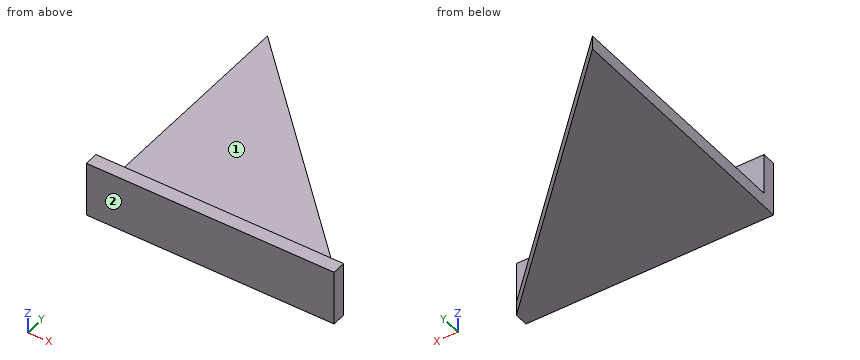
from build123d import *

# Parameters (mm, degrees)
F0_W     = 228.6
F0_H     = 50.8
F1_DEPTH = 12.7
F2_W     = 228.6
F2_H     = 12.7
F3_DEPTH = 228.6
F5_DEPTH = 25.4


with BuildPart() as f1:
    # F0 (on Front) → F1 (new body)
    with BuildSketch(Plane.XZ):
        Rectangle(F0_W, F0_H)
    extrude(amount=F1_DEPTH)

    # F2 (on face) → F3 (join)
    with BuildSketch(Plane(origin=(0, 0, 0), x_dir=(-1, 0, 0), z_dir=(0, 1, 0))):
        with Locations((0, -19.05)):
            Rectangle(F2_W, F2_H)
    extrude(amount=F3_DEPTH)

    # F4 (on face) → F5 (cut)
    with BuildSketch(Plane.XY.offset(-12.7)):
        Polygon((114.3, 228.6), (-114.3, 228.6), (114.3, 0), align=None)
    extrude(amount=-F5_DEPTH, mode=Mode.SUBTRACT)


solid = f1.part
Source: CAD feature listing. Evaluate the final solid. Frame: model axes, mm. Face numbers are marked on the shaded views. A direction names the side the tool comes from. Give positions to 0.01 mm unless a question says otherwise; leave off trailing zeros. Write each loop counter-clockwise with the first axis right and the second up, starting at its lowest first coordinate (ties: lowest second). Pieces come first, ordered by that corner, then holes. Notation, with made-up numbers: (28.25, 49.5) -> (75.25, 49.5) arc R23 ccw to (75.25, 59.5) -> close; hole circle Ø7 at (71.5, -19.75). An arc over 180 degrees is marked (long way). Return JSON: item names as keys, results as strings. Group by question number.
1. Section A-A, the plane x = -95.5. Output: boundary loops of the cut face in (y, z), then the cut area to 3 significant figures.
2. Section D-D, the plane x = -35. Output: boundary loops of the cut face in (y, z), then the cut area to 3 significant figures.
3. Section C-C, the plane z = -2.5. Output: boundary loops of the cut face in (x, y), then the cut area to 3 significant figures.
4. Pin query (flat end, axial travel): pin 1 Ø12 at (x, z) = (-56.5, 13.5) entering from +Y; pin 2 Ø10 at (y, z) = (115.5, -9.5) entering from -X; pin 3 Ø2 at (y, z) = (52.5, -11) entering from +X. Return the tip coordinate at first contact, or that it passes through.
5. Section B-B, the plane y = 99.5. Output: boundary loops of the cut face in (x, z), then the cut area to 3 significant figures.
6. Material intervals for line 1 (Y direction, x = 1.5, z = 13.5); line 2 (Z direction, x = 0.5, y = 31.5); line 3 (X direction, y = 141, z = -13.5), sorted ascending. Write a range as from..to.
7. Access query for the marked faces 1 and 2. Directions: +Z, -Z, +X, -X, +Y, -Y. A direction counts if a zero-diameter tool reaches every point of the face in a straight line with its end or side. Return the directions, or none.
Determined:
{
 "1": {"outline": "(-12.7, -25.4) -> (209.8, -25.4) -> (209.8, -12.7) -> (0, -12.7) -> (0, 25.4) -> (-12.7, 25.4) -> close", "area": "3,310 mm2"},
 "2": {"outline": "(-12.7, -25.4) -> (149.3, -25.4) -> (149.3, -12.7) -> (0, -12.7) -> (0, 25.4) -> (-12.7, 25.4) -> close", "area": "2,540 mm2"},
 "3": {"outline": "(-114.3, -12.7) -> (114.3, -12.7) -> (114.3, 0) -> (-114.3, 0) -> close", "area": "2,900 mm2"},
 "4": {"pin 1": "stops at y = 0", "pin 2": "stops at x = -114.3", "pin 3": "passes through"},
 "5": {"outline": "(-114.3, -25.4) -> (14.8, -25.4) -> (14.8, -12.7) -> (-114.3, -12.7) -> close", "area": "1,640 mm2"},
 "6": {"line 1": "y = -12.7..0", "line 2": "z = -25.4..-12.7", "line 3": "x = -114.3..-26.7"},
 "7": {"face 1": "+Z, +X, -X, +Y", "face 2": "+Z, -Z, +X, -X, -Y"}
}
